Can you work these out from the drawing? Everything is in mm from the part's minimum corner. A direction names the side the tool comes from. Coordinates: 2 decimals unless noted, no trailing zeros. Loops run counter-clockwise (first coordinate to the right, second up) from the corner with the lowest first, then second, coordinate; pieces in that order, holes last. Notation, with made-up numbers: (-36, 20) -> (-23, 20) arc R23 cw to (-23, 28) -> close; hole circle Ø11 at (66.5, 65). An arc over 180 degrees is marked (long way). Put each result on its own line as item: value. Start each with the question number.
Item 1: If we section it at D-D on y = 17.25: Please give me the cut outline in (x, z).
Item 2: If we section it at A-A on y = 14: Please give me the cut outline in (x, z), plus the area to 3 significant figures.
Item 3: If we section it at C-C on x = 8.25: Please give me the cut outline in (y, z).
Item 4: Please list where these lines run through material, in increasing order: L1, parallel to X at y = 13.75, z = 1.75; L2, parallel to X at y = 19, z = 5.5; L3, parallel to Y at x = 5.75, z = 6.5. Write a range as from..to.
Item 5: If we section it at B-B on z = 1.25: Please give me the cut outline in (x, y).
Item 6: Will these pins go through, and if not, where does the flat tip stop? P1, Ø1, axis at x = 22, z = 2.5, coming from the +Y side; P2, Ø2, axis at y = 12, z = 5, coming from the +X side; P3, Ø1, axis at x = 7, z = 2, coming from the +Y side.
Item 7: For the marked faces 4 and 5, which set-ups out of +Z, -Z, +X, -X, +Y, -Y let a thin tool reach every point of the face, with its end or its side?
Item 8: We'd pull the mould along X, two halves only. Please class the marked faces 1, 2 and 3: pulls with the +X half, pulls with the -X half, needs draft (parallel to the pull), parting line crosses it, or undercut.
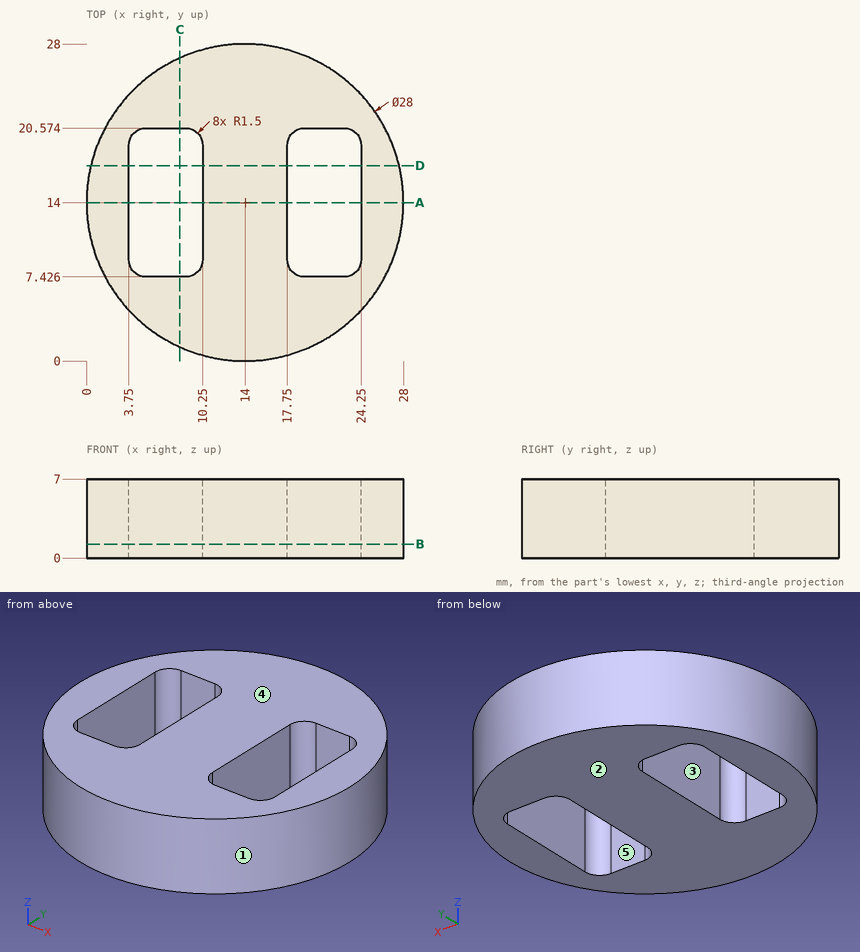
Solutions:
1. outline: (0.38, 0) -> (3.75, 0) -> (3.75, 7) -> (0.38, 7) -> close; (10.25, 0) -> (17.75, 0) -> (17.75, 7) -> (10.25, 7) -> close; (24.25, 0) -> (27.62, 0) -> (27.62, 7) -> (24.25, 7) -> close
2. outline: (0, 0) -> (3.75, 0) -> (3.75, 7) -> (0, 7) -> close; (10.25, 0) -> (17.75, 0) -> (17.75, 7) -> (10.25, 7) -> close; (24.25, 0) -> (28, 0) -> (28, 7) -> (24.25, 7) -> close
2. area: 105 mm^2
3. outline: (1.24, 0) -> (7.43, 0) -> (7.43, 7) -> (1.24, 7) -> close; (20.57, 0) -> (26.76, 0) -> (26.76, 7) -> (20.57, 7) -> close
4. L1: 0..3.75, 10.25..17.75, 24.25..28
4. L2: 0.92..3.75, 10.25..17.75, 24.25..27.08
4. L3: 2.69..7.43, 20.57..25.31
5. outline: circle Ø28 at (14, 14); hole (3.75, 8.93) arc R1.5 ccw to (5.25, 7.43) -> (8.75, 7.43) arc R1.5 ccw to (10.25, 8.93) -> (10.25, 19.07) arc R1.5 ccw to (8.75, 20.57) -> (5.25, 20.57) arc R1.5 ccw to (3.75, 19.07) -> close; hole (17.75, 8.93) arc R1.5 ccw to (19.25, 7.43) -> (22.75, 7.43) arc R1.5 ccw to (24.25, 8.93) -> (24.25, 19.07) arc R1.5 ccw to (22.75, 20.57) -> (19.25, 20.57) arc R1.5 ccw to (17.75, 19.07) -> close
6. P1: y = 25.82
6. P2: x = 27.96
6. P3: y = 26.4
7. face 4: +Z, +X, -X, +Y, -Y
7. face 5: +Z, -Z
8. face 1: parting line crosses it
8. face 2: needs draft
8. face 3: undercut
